The drawing under review shows one solid part. Ordinate dimensions are in mm from its lowest x, y, z. A direction names the side the tool comes from. Give positions to 0.01 mm unless a question says otherwise; leave off trailing zeros. Write each loop counter-clockwise with the first axis right and the second up, starting at its lowest first coordinate (ties: lowest second). Pieces come first, ordered by that corner, then holes. Notation, with made-up numbers: (-28, 52.5) - (19, 52.5) arc R23 ccw to (19, 73.5) - close; hole circle Ø10 at (-35, 24). An arc over 180 degrees is marked (long way). Write each question's results on one line, items separated by ' | '. Start each with the question number.
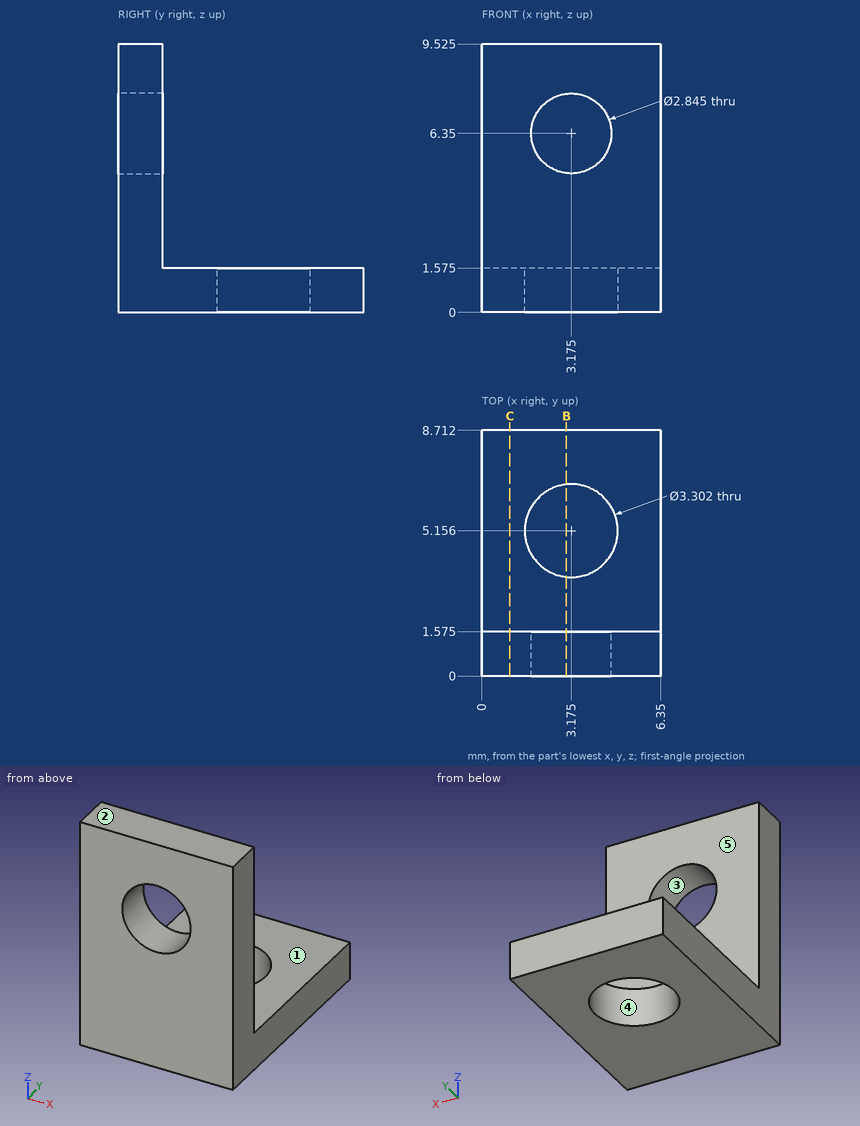
Q1. For line 1 along X through (y, z) = (0.7, 6.35); line 2 along Y through (x, z) = (3.25, 2.75) (1 decimal), list the stretches that pass through material, from the lowest coordinate up. Write a range as [from, to].
Q2. Insertion check: P1, Ø1.9, axis at x = 2.5, z = 3.5, coming from the +Y side (3 decimals). The pin has a flat end and moves straight along its axis. Give the tip position at first contact, or say it passes through.
Q3. The part is to be moulded in two halves that separate along Y. For the marked faces 3, 4 and 5, say which applies: +Y half, -Y half, draft (parallel to the pull), parting line (faces both ways), or undercut.
Q4. Machinability: for the marked faces 1 and 2, which of the approach directions +Z, -Z, +X, -X, +Y, -Y give a long, thin tool a straight path to every point of the face, cutting with its end or side? Answer none if there is none.
Q5. Add section C-C on x = 1. State the section outline as (y, z) points (1 decimal).
Q6. Add section B-B on x = 3. State the section outline as (y, z) points (1 decimal).
Result:
1) line 1: x = [0, 1.75], [4.6, 6.35] | line 2: y = [0, 1.6]
2) P1: stops at y = 1.575
3) face 3: draft | face 4: undercut | face 5: +Y half
4) face 1: +Z, +X, -X, +Y | face 2: +Z, +X, -X, +Y, -Y
5) outline: (0, 0) - (8.7, 0) - (8.7, 1.6) - (1.6, 1.6) - (1.6, 9.5) - (0, 9.5) - close
6) outline: (0, 0) - (3.5, 0) - (3.5, 1.6) - (1.6, 1.6) - (1.6, 4.9) - (0, 4.9) - close; (0, 7.8) - (1.6, 7.8) - (1.6, 9.5) - (0, 9.5) - close; (6.8, 0) - (8.7, 0) - (8.7, 1.6) - (6.8, 1.6) - close
